Geometry: final body of the model. Coordinates: model frame, mm. Give positions to 0.01 mm unless a question says otherwise; leave off trailing zeros. Loops run counter-clockwise (first coordinate to the right, second up) from the corner with the lowest first, then second, coordinate; pieces in that order, holes last. Notation, with made-up numbers: M -4.75,17.25 L 4.25,17.25 A21 ccw 4.25,31.25 Z; hole C 73,3 d3. An arc over 180 degrees is marked long. One line per question, with ' | ' between items. Start each with the question number.
from build123d import *

# Parameters (mm, degrees)
F0_R     = 76.841269309
F1_DEPTH = 25.4
F3_DEPTH = 2540
F4_DEPTH = 25.4


with BuildPart() as f1:
    # F0 (on Top) → F1 (new body)
    with BuildSketch(Plane.XY):
        Circle(F0_R)
        with BuildLine():
            ThreePointArc((49.1623187614, 22.610375279), (52.8604702506, 11.5729573203), (54.1125, 0))
            ThreePointArc((54.1125, 0), (52.8604702506, -11.5729573203), (49.1623187614, -22.610375279))
            Line((49.1623187614, -22.610375279), (58.0230537001, -27.7261229811))
            Line((58.0230537001, -27.7261229811), (53.0230537001, -36.3863770189))
            Line((53.0230537001, -36.3863770189), (44.1623187614, -31.2706293168))
            ThreePointArc((44.1623187614, -31.2706293168), (27.05625, -46.8627996623), (5, -53.8810045958))
            Line((5, -53.8810045958), (5, -64.1125))
            Line((5, -64.1125), (-5, -64.1125))
            Line((-5, -64.1125), (-5, -53.8810045958))
            ThreePointArc((-5, -53.8810045958), (-27.05625, -46.8627996623), (-44.1623187614, -31.2706293168))
            Line((-44.1623187614, -31.2706293168), (-53.0230537001, -36.3863770189))
            Line((-53.0230537001, -36.3863770189), (-58.0230537001, -27.7261229811))
            Line((-58.0230537001, -27.7261229811), (-49.1623187614, -22.610375279))
            ThreePointArc((-49.1623187614, -22.610375279), (-54.1125, 0), (-49.1623187614, 22.610375279))
            Line((-49.1623187614, 22.610375279), (-58.0230537001, 27.7261229811))
            Line((-58.0230537001, 27.7261229811), (-53.0230537001, 36.3863770189))
            Line((-53.0230537001, 36.3863770189), (-44.1623187614, 31.2706293168))
            ThreePointArc((-44.1623187614, 31.2706293168), (-27.05625, 46.8627996623), (-5, 53.8810045958))
            Line((-5, 53.8810045958), (-5, 64.1125))
            Line((-5, 64.1125), (5, 64.1125))
            Line((5, 64.1125), (5, 53.8810045958))
            ThreePointArc((5, 53.8810045958), (27.05625, 46.8627996623), (44.1623187614, 31.2706293168))
            Line((44.1623187614, 31.2706293168), (53.0230537001, 36.3863770189))
            Line((53.0230537001, 36.3863770189), (58.0230537001, 27.7261229811))
            Line((58.0230537001, 27.7261229811), (49.1623187614, 22.610375279))
        make_face(mode=Mode.SUBTRACT)
    extrude(amount=F1_DEPTH)

    # F2 (on face) → F3 (cut)
    with BuildSketch(Plane.XY.offset(25.4)):
        with BuildLine():
            Line((60.331269309, 0), (76.841269309, 0))
            ThreePointArc((76.841269309, 0), (76.8109087462, 2.1598533743), (76.7198510493, 4.318))
            Line((76.7198510493, 4.318), (71.6383990579, 4.318))
            Line((71.6383990579, 4.318), (66.681269309, 4.318))
            Line((66.681269309, 4.318), (66.681269309, 10.16))
            Line((66.681269309, 10.16), (60.331269309, 10.16))
            Line((60.331269309, 10.16), (60.331269309, 0))
        make_face()
        with BuildLine():
            Line((66.681269309, -4.318), (71.6383990579, -4.318))
            Line((71.6383990579, -4.318), (76.7198510493, -4.318))
            ThreePointArc((76.7198510493, -4.318), (76.8109087462, -2.1598533743), (76.841269309, 0))
            Line((76.841269309, 0), (60.331269309, 0))
            Line((60.331269309, 0), (60.331269309, -10.16))
            Line((60.331269309, -10.16), (66.681269309, -10.16))
            Line((66.681269309, -10.16), (66.681269309, -4.318))
        make_face()
    extrude(amount=-F3_DEPTH, mode=Mode.SUBTRACT)

    # F2 (on face) → F4 (join)
    with BuildSketch(Plane.XY.offset(25.4)):
        with BuildLine():
            Line((81.0480539402, 8.8309641961), (69.4320089527, 32.9207655108))
            ThreePointArc((69.4320089527, 32.9207655108), (72.3316680057, 25.93666271), (74.5307966821, 18.7013639864))
            add(Edge.make_bspline(
                [(74.5307966821, 18.7013639864), (75.9347240562, 15.3777124362), (77.4050082281, 12.5783342613), (78.9966583252, 10.7205696404)],
                knots=[0.3571653837, 0.3571653837, 0.3571653837, 0.3571653837, 0.6407462723, 0.6407462723, 0.6407462723, 0.6407462723], degree=3))
            add(Edge.make_bspline(
                [(78.9966583252, 10.7205696404), (79.6616242514, 9.944425327), (80.3477738062, 9.3326335024), (81.0480539402, 8.8309641961)],
                knots=[0.6407462723, 0.6407462723, 0.6407462723, 0.6407462723, 0.759221827, 0.759221827, 0.759221827, 0.759221827], degree=3))
        make_face()
        with BuildLine():
            add(Edge.make_bspline(
                [(74.5307966821, 18.7013639864), (75.9347240562, 15.3777124362), (77.4050082281, 12.5783342613), (78.9966583252, 10.7205696404)],
                knots=[0.3571653837, 0.3571653837, 0.3571653837, 0.3571653837, 0.6407462723, 0.6407462723, 0.6407462723, 0.6407462723], degree=3))
            ThreePointArc((74.5307966821, 18.7013639864), (75.4668021106, 14.4686712665), (76.1626284874, 10.1899308588))
            Line((76.1626284874, 10.1899308588), (78.9966583252, 10.7205696404))
        make_face()
        with BuildLine():
            ThreePointArc((76.1626284874, 10.1899308588), (76.4976014678, 7.2593139274), (76.7198510493, 4.318))
            Line((76.7198510493, 4.318), (76.841269309, 4.318))
            Line((76.841269309, 4.318), (83.2241945586, 4.318))
            Line((83.2241945586, 4.318), (78.9966583252, 10.7205696404))
            Line((78.9966583252, 10.7205696404), (76.1626284874, 10.1899308588))
        make_face()
        with BuildLine():
            Line((83.2241945586, 4.318), (81.0480539402, 8.8309641961))
            add(Edge.make_bspline(
                [(78.9966583252, 10.7205696404), (79.6616242514, 9.944425327), (80.3477738062, 9.3326335024), (81.0480539402, 8.8309641961)],
                knots=[0.6407462723, 0.6407462723, 0.6407462723, 0.6407462723, 0.759221827, 0.759221827, 0.759221827, 0.759221827], degree=3))
            Line((78.9966583252, 10.7205696404), (83.2241945586, 4.318))
        make_face()
        with BuildLine():
            ThreePointArc((76.7198510493, -4.318), (76.4976014678, -7.2593139274), (76.1626284874, -10.1899308588))
            Line((76.1626284874, -10.1899308588), (78.9966583252, -10.7205696404))
            add(Edge.make_bspline(
                [(78.9966583252, -10.7205696404), (79.6616242514, -9.944425327), (80.3477738062, -9.3326335024), (81.0480539402, -8.8309641961)],
                knots=[0.6407462723, 0.6407462723, 0.6407462723, 0.6407462723, 0.759221827, 0.759221827, 0.759221827, 0.759221827], degree=3))
            Line((81.0480539402, -8.8309641961), (83.2241945586, -4.318))
            Line((83.2241945586, -4.318), (76.841269309, -4.318))
            Line((76.841269309, -4.318), (76.7198510493, -4.318))
        make_face()
        with BuildLine():
            add(Edge.make_bspline(
                [(78.9966583252, -10.7205696404), (79.6616242514, -9.944425327), (80.3477738062, -9.3326335024), (81.0480539402, -8.8309641961)],
                knots=[0.6407462723, 0.6407462723, 0.6407462723, 0.6407462723, 0.759221827, 0.759221827, 0.759221827, 0.759221827], degree=3))
            add(Edge.make_bspline(
                [(74.5307966821, -18.7013639864), (75.9347240562, -15.3777124362), (77.4050082281, -12.5783342613), (78.9966583252, -10.7205696404)],
                knots=[0.3571653837, 0.3571653837, 0.3571653837, 0.3571653837, 0.6407462723, 0.6407462723, 0.6407462723, 0.6407462723], degree=3))
            ThreePointArc((74.5307966821, -18.7013639864), (72.3316680057, -25.93666271), (69.4320089527, -32.9207655108))
            Line((69.4320089527, -32.9207655108), (81.0480539402, -8.8309641961))
        make_face()
        with BuildLine():
            Line((78.9966583252, -10.7205696404), (76.1626284874, -10.1899308588))
            ThreePointArc((76.1626284874, -10.1899308588), (75.4668021106, -14.4686712665), (74.5307966821, -18.7013639864))
            add(Edge.make_bspline(
                [(74.5307966821, -18.7013639864), (75.9347240562, -15.3777124362), (77.4050082281, -12.5783342613), (78.9966583252, -10.7205696404)],
                knots=[0.3571653837, 0.3571653837, 0.3571653837, 0.3571653837, 0.6407462723, 0.6407462723, 0.6407462723, 0.6407462723], degree=3))
        make_face()
    extrude(amount=-F4_DEPTH)


solid = f1.part
Q1. Section B-B, the plane y = 57. Output: boundary loops of the cut face in (x, z), plus the area to 3 significant figures.
Q2. Contact query for flat-ended pins moving along their axis: pin 1 (3 mm diameter, centred on y = -44.5, z = 14, fed in from +X); pin 2 (8 mm diameter, centred on y = -58.5, z = 12.5, fed in from -X); pin 3 (5 mm diameter, centred on x = 73, z = 7, fed in from +Y). Output: stop coordinate, or through.
Q3. Draft query along Y for faces 1 (the flat face through (75, -4.318, 13)), 2 (the flat face through (75, 4.318, 13)). Return one class per face: released by +Y, released by -Y, zero draft, split by the parting line, or undercut.
Q4. Section A-A, the plane x = 0. Output: boundary loops of the cut face in (y, z), plus the area to 3 significant figures.
Q5. Section C-C, the plane y = -66. Output: boundary loops of the cut face in (x, z), plus the area to 3 significant figures.
Q6. Material intervals for L1, parallel to X at y = 1.5, z = 13.25; L2, parallel to Y at x = -55, z = 18.25; L3, parallel to Y at x = 73, z = 12.75, sorted ascending.
Model answer:
1) outline: M -51.53,0 L -5,0 L -5,25.4 L -51.53,25.4 Z; M 5,0 L 51.53,0 L 51.53,25.4 L 5,25.4 Z | area: 2,360 mm^2
2) pin 1: stops at x = 63.68 | pin 2: stops at x = -54.17 | pin 3: stops at y = 30.71
3) face 1: undercut | face 2: undercut
4) outline: M -76.84,0 L -64.11,0 L -64.11,25.4 L -76.84,25.4 Z; M 64.11,0 L 76.84,0 L 76.84,25.4 L 64.11,25.4 Z | area: 647 mm^2
5) outline: M -39.35,0 L 39.35,0 L 39.35,25.4 L -39.35,25.4 Z | area: 2,000 mm^2
6) L1: x = -76.83 to -54.09, 54.09 to 60.33 | L2: y = -53.66 to -32.96, -25.98 to 25.98, 32.96 to 53.66 | L3: y = -25.52 to -4.32, 4.32 to 25.52
